```python
from build123d import *

# Parameters (mm, degrees)
BOSS_EXTRUDE1_DEPTH      = 12
SKETCH2_R                = 1
CUT_EXTRUDE1_DEPTH       = 13.592987467
CHAMFER1_SIZE            = 0.1
BOSS_EXTRUDE2_DEPTH      = 2.7
BOSS_EXTRUDE2_DEPTH_BACK = 2.7
SKETCH3_R                = 1.2


with BuildPart() as part:
    # Sketch1 → Boss-Extrude1 (new body)
    with BuildSketch(Plane(origin=(0, 0, 0), x_dir=(1, 0, 0), z_dir=(0, 1, 0))):
        Polygon((0, 2.886751346), (-2.5, 1.443375673), (-2.5, -1.443375673), (0, -2.886751346), (2.5, -1.443375673), (2.5, 1.443375673), align=None)
    extrude(amount=BOSS_EXTRUDE1_DEPTH)

    # Sketch2 → Cut-Extrude1 (cut, through all)
    with BuildSketch(Plane(origin=(0, 12, 0), x_dir=(1, 0, 0), z_dir=(0, 1, 0))):
        with Locations(Location((0, 0, 0), (0, 0, 270))):
            Circle(SKETCH2_R)
    extrude(amount=-CUT_EXTRUDE1_DEPTH, mode=Mode.SUBTRACT)

    # Chamfer1
    chamfer1_edges = [part.edges().sort_by_distance(p)[0] for p in [
        (-2.5, 12, 0),
        (-1.25, 12, 2.165063509),
        (1.25, 12, 2.165063509),
        (2.5, 12, 0),
        (0, 12, -1),
        (1.25, 12, -2.165063509),
        (2.5, 0, 0),
        (1.25, 0, 2.165063509),
        (-1.25, 0, 2.165063509),
        (-1.25, 12, -2.165063509),
        (-2.5, 0, 0),
        (-1.25, 0, -2.165063509),
        (1.25, 0, -2.165063509),
    ]]
    chamfer(chamfer1_edges, length=CHAMFER1_SIZE)

    # Sketch3 → Boss-Extrude2 (add, two sides: drawn at the far end of the back side and taken through both)
    with BuildSketch(Plane.XZ.offset(-BOSS_EXTRUDE2_DEPTH_BACK)):
        with Locations(Location((0, 0, 0), (0, 0, 270))):
            Circle(SKETCH3_R)
    extrude(amount=BOSS_EXTRUDE2_DEPTH + BOSS_EXTRUDE2_DEPTH_BACK)


solid = part.part
```
Model file for the job. Use its own axes, mm. A direction names the side the tool comes from. Round coordinates to 2 decimals unless told otherwise and drop trailing zeros. Loops run counter-clockwise (first coordinate to the right, second up) from the corner with the lowest first, then second, coordinate; pieces in that order, holes last. Notation, with made-up numbers: M -29.5,22 L -2.5,22 A24 ccw -2.5,35 Z; hole C -27,67 d6. An arc over 180 degrees is marked long. Put each result on its own line as item: value. Start each with the question number.
Item 1: Drop flat-ended pins along their axis: P1, Ø0.6, axis at x = 0.5, z = 0, coming from the +Y side; P2, Ø2, axis at x = -0.5, y = 9, coming from the -Z side. Give the stop position or say it passes through.
Item 2: Cut at D-D (x = 1.8). List the corners of the cut face in (y, z).
Item 3: 3-axis set-ups, long thin cutter, end or side, ignore diameter. For faces 1 (the face through (2.5, 6, 0)), 2 (the face through (-1, 7, 0)), 3 (the face through (1.01, -1.33, -0.65)): which of +Z, -Z, +X, -X, +Y, -Y reach the whole face in a straight line?
Item 4: Cut at B-B (z = 0). List the corners of the cut face in (x, y), then the cut area to 4 significant figures.
Item 5: Cut at A-A (y = 9.75). List the corners of the cut face in (x, z).
Item 6: Cut at C-C (y = 1.25). List the corners of the cut face in (x, z).
Item 7: Mould opens along Z. For faces 4 (the face through (0, 2.7, 0)), 5 (the face through (1.267, 5.917, -2.155)), 6 (the face through (-1, 0, 1)) say: released by +Z, released by -Z, zero draft, split by the parting line, or undercut.
Item 8: Drill centre lines: line 1 along X through (y, z) = (9.5, 0); line 2 along Y through (x, z) = (1.15, -0.45); line 3 along X through (y, z) = (10.5, -2.25). Where is each one in solid material? Low to high.
Answer block:
1. P1: y = 2.7
1. P2: z = -2.89
2. outline: M 0,-1.73 L 0.1,-1.85 L 11.9,-1.85 L 12,-1.73 L 12,1.73 L 11.9,1.85 L 0.1,1.85 L 0,1.73 Z
3. face 1: +Z, -Z, +X, +Y, -Y
3. face 2: +Y
3. face 3: -Y
4. outline: M -2.5,0.1 L -2.4,0 L -1.2,0 L -1.2,-2.7 L 1.2,-2.7 L 1.2,0 L 2.4,0 L 2.5,0.1 L 2.5,11.9 L 2.4,12 L 1.1,12 L 1,11.9 L 1,2.7 L -1,2.7 L -1,11.9 L -1.1,12 L -2.4,12 L -2.5,11.9 Z
4. area: 47.85 mm2
5. outline: M -2.5,-1.44 L 0,-2.89 L 2.5,-1.44 L 2.5,1.44 L 0,2.89 L -2.5,1.44 Z; hole C 0,0 d2
6. outline: M -2.5,-1.44 L 0,-2.89 L 2.5,-1.44 L 2.5,1.44 L 0,2.89 L -2.5,1.44 Z
7. face 4: undercut
7. face 5: released by -Z
7. face 6: zero draft
8. line 1: -2.5 to -1, 1 to 2.5
8. line 2: 0 to 12
8. line 3: -1.1 to 1.1
